The drawing under review shows one solid part. Ordinate dimensions are in mm from its lowest x, y, z. A direction names the side the tool comes from. Round coordinates to 2 decimals unless told otherwise and drop trailing zeros. Write each loop counter-clockwise with the first axis right and the second up, starting at its lowest first coordinate (ties: lowest second). Pieces come first, ordered by that corner, then holes. Notation, with made-up numbers: M 55,63.25 L 92,63.25 A31 ccw 92,100.25 Z; hole C 34,30 d3. An arc over 180 degrees is marked long. One line per item, written item: value. Start each with the question number.
1) Take a section at B-B, the plane x = 4. Write out the cut boundary in (y, z).
2) Take a section at D-D, the plane y = 0.8. Write out the cut boundary in (x, z), and give its area (3 significant figures).
3) Wall thickness on probe 1 along Z at (x, y) = (2, 1.45); probe 2 along Z at (x, y) = (3.25, 2.05); probe 3 along Y at (x, z) = (4.5, 24.5): over which ranges is each line inside the solid? List them lowest first.
4) Take a section at A-A, the plane y = 2.7. Write out the cut boundary in (x, z), and give its area (3 significant figures).
5) For P1, Ø1, axis at y = 4.5, z = 8.5, coming from the -X side; P2, Ø1.5, axis at y = 2.5, z = 15.5, coming from the -X side; P3, Ø1, axis at x = 2.5, y = 4, coming from the -Z side; P4, Ø1.1, axis at y = 2.5, z = 2.5, coming from the +X side, all flat-tipped, find the tip position at first contact; note any pin that passes through.
6) Take a section at C-C, the plane z = 23.75. Write out the cut boundary in (x, y), and give its area (3 significant figures).
7) Tool access review of the marked faces 1 and 2: name each direction out of +Z, -Z, +X, -X, +Y, -Y from which nothing blocks a thin tool from reaching the whole face with its end or side.
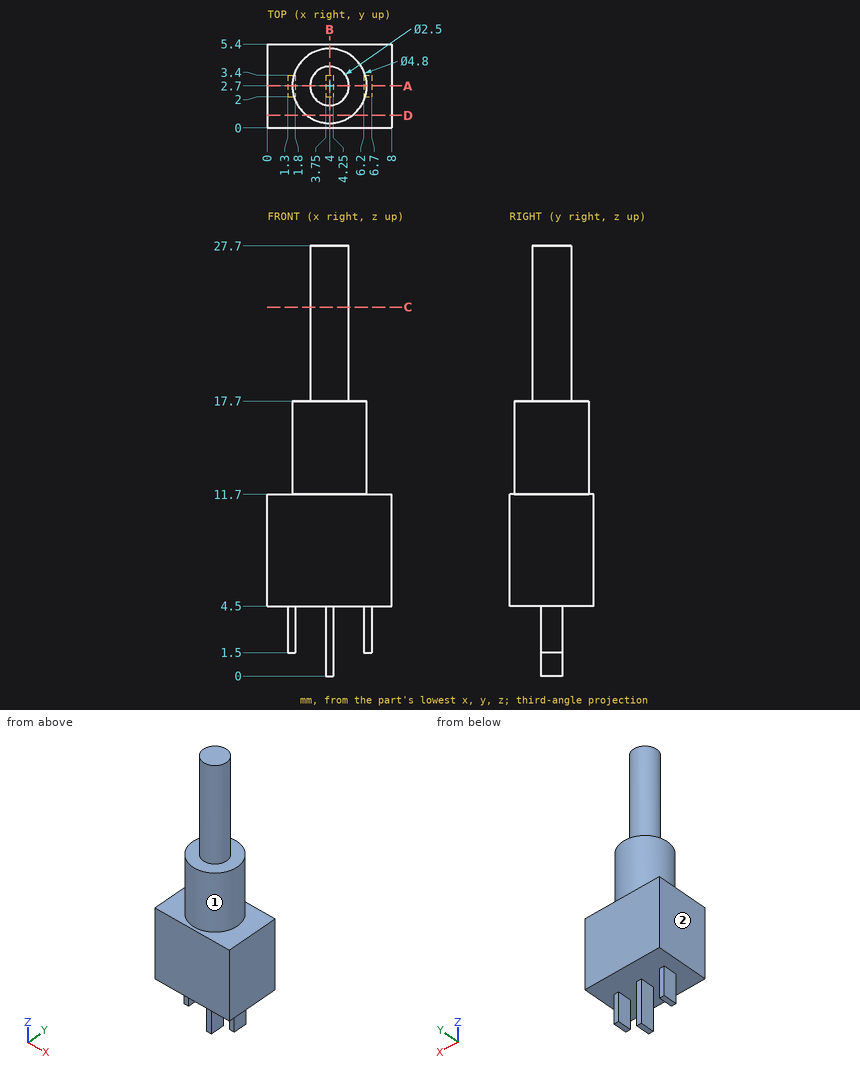
Checked values:
1. outline: M 0,4.5 L 2,4.5 L 2,0 L 3.4,0 L 3.4,4.5 L 5.4,4.5 L 5.4,11.7 L 5.1,11.7 L 5.1,17.7 L 3.95,17.7 L 3.95,27.7 L 1.45,27.7 L 1.45,17.7 L 0.3,17.7 L 0.3,11.7 L 0,11.7 Z
2. outline: M 0,4.5 L 8,4.5 L 8,11.7 L 5.47,11.7 L 5.47,17.7 L 2.53,17.7 L 2.53,11.7 L 0,11.7 Z
2. area: 75.2 mm2
3. probe 1: z = 4.5 to 17.7
3. probe 2: z = 4.5 to 27.7
3. probe 3: y = 1.55 to 3.85
4. outline: M 0,4.5 L 1.3,4.5 L 1.3,1.5 L 1.8,1.5 L 1.8,4.5 L 3.75,4.5 L 3.75,0 L 4.25,0 L 4.25,4.5 L 6.2,4.5 L 6.2,1.5 L 6.7,1.5 L 6.7,4.5 L 8,4.5 L 8,11.7 L 6.4,11.7 L 6.4,17.7 L 5.25,17.7 L 5.25,27.7 L 2.75,27.7 L 2.75,17.7 L 1.6,17.7 L 1.6,11.7 L 0,11.7 Z
4. area: 117 mm2
5. P1: stops at x = 0
5. P2: stops at x = 1.6
5. P3: stops at z = 4.5
5. P4: stops at x = 6.7
6. outline: C 4,2.7 d2.5
6. area: 4.91 mm2
7. face 1: +Z
7. face 2: +Z, -Z, -X, +Y, -Y
